Could you check a few things on this model? Use its own coordinates, in mm. A direction names the side the tool comes from. Coordinates: 2 decimals unless noted, no trailing zeros. Loops run counter-clockwise (first coordinate to the right, second up) from the corner with the lowest first, then second, coordinate; pieces in that order, holes last.
1) Imagine slicing it at A-A on x = -7. Please give me the cut outline in (y, z), plus the area to 3 significant figures.
2) If I drill on line 1 along Z through (x, y) = (-6.5, 6.25); line 2 along X through (y, z) = (4.2, -22.45); line 3 along Z through (x, y) = (11, 12.75), over which ranges is the centre line in solid material (lowest first)?
3) Thinking about a two-plate mould opening in X: for faces 1 (the face through (-26.476, 4.535, -23.391)), 2 (the face through (-23.524, 4.535, 23.391)), 3 (the face through (8, 13, 27)), 4 (the face through (-30, 4, 22)), which applies, released by +X, released by -X, zero draft, split by the parting line, or undercut?
4) Will these pins go through, and if not, where does the flat tip stop? P1, Ø3, axis at x = -11, y = 9.5, coming from the +Z side; P2, Ø2.5, axis at x = -9.5, z = -21.5, coming from the +Y side; P3, Ø16.5, axis at x = 10.5, z = -4.5, coming from the +Y side; P4, Ø5, axis at y = 10, z = 19, coming from the -X side.
5) Imagine slicing it at B-B on x = -25. Please give me the cut outline in (y, z), plus the area to 3 significant figures.
6) Imagine slicing it at C-C on z = -22.45. Please give me the cut outline in (x, y), plus the area to 4 significant figures.
7) For faces 5 (the face through (-15, 2, -22)), 6 (the face through (7, 12, -19.95)), 7 (the face through (8, 7, -29)), 8 (the face through (8, 7, 29)), 9 (the face through (-15, 7, -22)), which set-ups out of +Z, -Z, +X, -X, +Y, -Y let a thin tool reach every point of the face, with its end or its side?
8) Imagine slicing it at D-D on x = 3. Please give me the cut outline in (y, z), plus the area to 3 significant figures.
```python
from build123d import *

# Parameters (mm, degrees)
SKETCH1_W           = 15
SKETCH1_H           = 49.9
BOSS_EXTRUDE1_DEPTH = 2
SKETCH2_W           = 45
SKETCH2_H           = 5
BOSS_EXTRUDE2_DEPTH = 5
SKETCH3_R           = 1.75
CUT_EXTRUDE1_DEPTH  = 40.642180818
SKETCH4_W           = 15
SKETCH4_H           = 49.9
BOSS_EXTRUDE3_DEPTH = 13
SKETCH5_W           = 15
SKETCH5_H           = 6
BOSS_EXTRUDE4_DEPTH = 10
SKETCH6_R           = 1.75
CUT_EXTRUDE2_DEPTH  = 48.859194519
SKETCH7_W           = 15
SKETCH7_H           = 39.9
CUT_EXTRUDE3_DEPTH  = 2.5


with BuildPart() as part:
    # Sketch1 → Boss-Extrude1 (new body)
    with BuildSketch(Plane(origin=(0, 0, 0), x_dir=(1, 0, 0), z_dir=(0, 1, 0))):
        with Locations((7.5, 0)):
            Rectangle(SKETCH1_W, SKETCH1_H)
    extrude(amount=BOSS_EXTRUDE1_DEPTH)

    # Sketch2 → Boss-Extrude2 (add)
    with BuildSketch(Plane(origin=(0, 2, 0), x_dir=(1, 0, 0), z_dir=(0, 1, 0))):
        with Locations((-7.5, -22.45)):
            Rectangle(SKETCH2_W, SKETCH2_H)
        with Locations((-7.5, 22.45)):
            Rectangle(SKETCH2_W, SKETCH2_H)
    extrude(amount=BOSS_EXTRUDE2_DEPTH)

    # Sketch3 → Cut-Extrude1 (cut, through all)
    with BuildSketch(Plane(origin=(0, 7, 0), x_dir=(1, 0, 0), z_dir=(0, 1, 0))):
        with Locations(Location((-25, -22.45, 0), (0, 0, 270))):
            Circle(SKETCH3_R)
        with Locations(Location((-25, 22.45, 0), (0, 0, 90))):
            Circle(SKETCH3_R)
    extrude(amount=-CUT_EXTRUDE1_DEPTH, mode=Mode.SUBTRACT)

    # Sketch4 → Boss-Extrude3 (add)
    with BuildSketch(Plane(origin=(0, 0, 0), x_dir=(1, 0, 0), z_dir=(0, 1, 0))):
        with Locations((7.5, 0)):
            Rectangle(SKETCH4_W, SKETCH4_H)
    extrude(amount=BOSS_EXTRUDE3_DEPTH)

    # Sketch5 → Boss-Extrude4 (add)
    with BuildSketch(Plane(origin=(0, 0, -24.95), x_dir=(-1, 0, 0), z_dir=(0, 0, -1))):
        with Locations((-7.5, 10)):
            Rectangle(SKETCH5_W, SKETCH5_H)
    boss_extrude4 = extrude(amount=BOSS_EXTRUDE4_DEPTH)

    # Sketch6 → Cut-Extrude2 (cut, through all)
    with BuildSketch(Plane(origin=(0, 13, 0), x_dir=(1, 0, 0), z_dir=(0, 1, 0))):
        with Locations(Location((7.722564817, 30.885688998, 0), (0, 0, 270))):
            Circle(SKETCH6_R)
    cut_extrude2 = extrude(amount=-CUT_EXTRUDE2_DEPTH, mode=Mode.SUBTRACT)

    # Mirror1: Boss-Extrude4, Cut-Extrude2 across plane
    add(boss_extrude4.mirror(Plane.XY))
    add(cut_extrude2.mirror(Plane.XY), mode=Mode.SUBTRACT)

    # Sketch7 → Cut-Extrude3 (cut)
    with BuildSketch(Plane(origin=(0, 13, 0), x_dir=(1, 0, 0), z_dir=(0, 1, 0))):
        with Locations((7.5, 0)):
            Rectangle(SKETCH7_W, SKETCH7_H)
    extrude(amount=-CUT_EXTRUDE3_DEPTH, mode=Mode.SUBTRACT)


solid = part.part
```
Filled in:
1. outline: (2, -24.95) - (7, -24.95) - (7, -19.95) - (2, -19.95) - close; (2, 19.95) - (7, 19.95) - (7, 24.95) - (2, 24.95) - close
1. area: 50.0 mm2
2. line 1: z = -24.95 to -19.95, 19.95 to 24.95
2. line 2: x = -30 to -26.75, -23.25 to 15
2. line 3: z = -34.95 to -19.95, 19.95 to 34.95
3. face 1: undercut
3. face 2: undercut
3. face 3: zero draft
3. face 4: released by -X
4. P1: passes through
4. P2: stops at y = 7
4. P3: stops at y = 10.5
4. P4: stops at x = 0
5. outline: (2, -24.95) - (7, -24.95) - (7, -24.2) - (2, -24.2) - close; (2, -20.7) - (7, -20.7) - (7, -19.95) - (2, -19.95) - close; (2, 19.95) - (7, 19.95) - (7, 20.7) - (2, 20.7) - close; (2, 24.2) - (7, 24.2) - (7, 24.95) - (2, 24.95) - close
5. area: 15.0 mm2
6. outline: (-30, 2) - (-26.75, 2) - (-26.75, 7) - (-30, 7) - close; (-23.25, 2) - (0, 2) - (0, 0) - (15, 0) - (15, 13) - (0, 13) - (0, 7) - (-23.25, 7) - close
6. area: 327.5 mm2
7. face 5: +Z, -Z, -X, -Y
7. face 6: +X, -X, +Y
7. face 7: -Z, +X, -X, -Y
7. face 8: +Z, +X, -X, -Y
7. face 9: +Z, -Z, -X, +Y
8. outline: (0, -24.95) - (7, -24.95) - (7, -34.95) - (13, -34.95) - (13, -19.95) - (10.5, -19.95) - (10.5, 19.95) - (13, 19.95) - (13, 34.95) - (7, 34.95) - (7, 24.95) - (0, 24.95) - close
8. area: 669 mm2
